For this review, take the finished solid that the model builds, in its own axes (mm). A direction names the side the tool comes from. Give positions to 0.01 mm unless a question says otherwise; leave off trailing zeros. Write each loop counter-clockwise with the first axis right and the second up, starting at its lowest first coordinate (ties: lowest second). Pieces come first, ordered by that corner, then holes. Notation, with made-up numbers: (71.5, 84.5) -> (111.5, 84.5) arc R14 cw to (111.5, 93.5) -> close; hole circle Ø5 at (-32.5, 77). An arc over 180 degrees is marked (long way). Return JSON: item names as keys, results as strings.
from build123d import *

# Parameters (mm, degrees)
SKETCH1_W                                        = 71
SKETCH1_H                                        = 46
SKETCH1_W_2                                      = 32
SKETCH1_H_2                                      = 26
BOSS_EXTRUDE1_DEPTH                              = 7
SKETCH1_2_W                                      = 32
SKETCH1_2_H                                      = 26
BOSS_EXTRUDE2_DEPTH                              = 3
CBORE_FOR_M3_HEX_HEAD_MACHINE_SCREW1_D           = 3.4
CBORE_FOR_M3_HEX_HEAD_MACHINE_SCREW1_CBORE_D     = 8.4
CBORE_FOR_M3_HEX_HEAD_MACHINE_SCREW1_CBORE_DEPTH = 2.3
SKETCH6_W                                        = 4
SKETCH6_H                                        = 10.5
CUT_EXTRUDE1_DEPTH                               = 43.488233665
FILLET1_R                                        = 2


with BuildPart() as part:
    # Sketch1 → Boss-Extrude1 (new body)
    with BuildSketch(Plane(origin=(0, 0, 0), x_dir=(1, 0, 0), z_dir=(0, 1, 0))):
        Rectangle(SKETCH1_W, SKETCH1_H)
        with Locations((-17.5, 8)):
            Rectangle(SKETCH1_W_2, SKETCH1_H_2, mode=Mode.SUBTRACT)
        with Locations((17.5, 8)):
            Rectangle(SKETCH1_W_2, SKETCH1_H_2, mode=Mode.SUBTRACT)
    extrude(amount=BOSS_EXTRUDE1_DEPTH)

    # Sketch1<2> → Boss-Extrude2 (add)
    with BuildSketch(Plane(origin=(0, 0, 0), x_dir=(1, 0, 0), z_dir=(0, 1, 0))):
        with Locations((-17.5, 8)):
            Rectangle(SKETCH1_2_W, SKETCH1_2_H)
        with Locations((17.5, 8)):
            Rectangle(SKETCH1_2_W, SKETCH1_2_H)
    extrude(amount=BOSS_EXTRUDE2_DEPTH)

    # CBORE for M3 Hex Head Machine Screw1 (through all)
    with Locations(Plane(origin=(0, 7, 0), x_dir=(1, 0, 0), z_dir=(0, 1, 0))):
        with Locations((-23, -17), (23, -17)):
            CounterBoreHole(CBORE_FOR_M3_HEX_HEAD_MACHINE_SCREW1_D / 2, CBORE_FOR_M3_HEX_HEAD_MACHINE_SCREW1_CBORE_D / 2, CBORE_FOR_M3_HEX_HEAD_MACHINE_SCREW1_CBORE_DEPTH)

    # Sketch6 → Cut-Extrude1 (cut, through all)
    with BuildSketch(Plane(origin=(0, 3, 0), x_dir=(1, 0, 0), z_dir=(0, 1, 0))):
        with Locations((-31.5, 8)):
            Rectangle(SKETCH6_W, SKETCH6_H)
        with Locations((-3.5, 8)):
            Rectangle(SKETCH6_W, SKETCH6_H)
        with Locations((3.5, 8)):
            Rectangle(SKETCH6_W, SKETCH6_H)
        with Locations((31.5, 8)):
            Rectangle(SKETCH6_W, SKETCH6_H)
    extrude(amount=-CUT_EXTRUDE1_DEPTH, mode=Mode.SUBTRACT)

    # Fillet1
    fillet1_edges = [part.edges().sort_by_distance(p)[0] for p in [
        (-35.5, 7, 0),
        (35.5, 7, 0),
        (0, 7, -23),
    ]]
    fillet(fillet1_edges, radius=FILLET1_R - 0.0001)  # a hair under: the kernel refuses the full size


solid = part.part
1. For pin 1 (1.5 mm diameter, centred on y = 6, z = 12, fed in from -X); pin 2 (2.5 mm diameter, centred on x = -23, z = 17, fed in from +Y); pin 3 (5 mm diameter, centred on x = 5.5, z = -7, fed in from +Y); pin 4 (5 mm diameter, centred on x = -23, z = 17, fed in from +Y), all flat-tipped, find the tip position at first contact; note any pin that passes through.
Results found:
{"pin 1": "stops at x = -35.48", "pin 2": "passes through", "pin 3": "stops at y = 3", "pin 4": "stops at y = 4.7"}
2. To check wall thickness, follow probe 1 along X at (y, z) = (1.1, 17); probe 2 along X at (y, z) = (1, -6); probe 3 along Z at (x, y) = (23, 3.55). State the ranges of each line that lie inside material, in increasing order.
Results found:
{"probe 1": "x = -35.5 to -24.7, -21.3 to 21.3, 24.7 to 35.5", "probe 2": "x = -35.5 to -33.5, -29.5 to -5.5, -1.5 to 1.5, 5.5 to 29.5, 33.5 to 35.5", "probe 3": "z = -23 to -21, 5 to 15.3, 18.7 to 23"}
3. Add section A-A, the plane y = 4. State the section outline as (x, z) points, plus the area to 3 significant figures.
Results found:
{"outline": "(-35.5, -23) -> (35.5, -23) -> (35.5, 23) -> (-35.5, 23) -> close; hole (-33.5, -21) -> (-1.5, -21) -> (-1.5, 5) -> (-33.5, 5) -> close; hole circle Ø3.4 at (-23, 17); hole (1.5, -21) -> (33.5, -21) -> (33.5, 5) -> (1.5, 5) -> close; hole circle Ø3.4 at (23, 17)", "area": "1,580 mm²"}
4. The part is to be moulded in two halves that separate along X. For faces 4 (the cylindrical face through (-34.93, 6.4, -0.32)), 5 (the cylindrical face through (-24.57, 2.32, 17.65)), 6 (the flat face through (0, 2, -23)), say which applies: +X half, -X half, draft (parallel to the pull), parting line (faces both ways), or undercut.
Results found:
{"face 4": "-X half", "face 5": "undercut", "face 6": "draft"}
5. Add section D-D, the plane z = -6. Count the separate pieces of the cut face and the enclosed holes in it, plus the area to 3 significant figures.
Results found:
{"separate pieces": "5", "enclosed holes": "0", "area": "191 mm²"}
6. For faces 1 (the flat face through (35.5, 2, 0)), 2 (the flat face through (17, 5, -21)), 3 (the flat face through (-4, 2, -13.25)), list the 3-axis set-ups (+Z, -Z, +X, -X, +Y, -Y) from which the entire face can be reached by the end or side of a thin tool; tool diameter is ignored.
Results found:
{"face 1": "+Z, -Z, +X, +Y, -Y", "face 2": "+Y", "face 3": "+Y, -Y"}
7. Add section C-C, the plane z = 17. State the section outline as (x, y) points.
Results found:
{"outline": "(-35.5, 0) -> (-24.7, 0) -> (-24.7, 4.7) -> (-27.2, 4.7) -> (-27.2, 7) -> (-33.5, 7) arc R2 ccw to (-35.5, 5) -> close; (-21.3, 0) -> (21.3, 0) -> (21.3, 4.7) -> (18.8, 4.7) -> (18.8, 7) -> (-18.8, 7) -> (-18.8, 4.7) -> (-21.3, 4.7) -> close; (24.7, 0) -> (35.5, 0) -> (35.5, 5) arc R2 ccw to (33.5, 7) -> (27.2, 7) -> (27.2, 4.7) -> (24.7, 4.7) -> close"}
